Design review of the part shown in the three views and the two pictorial views. Dimensions are in mm from the part's minimum x, y and z. Coordinates: 2 decimals unless noted, no trailing zeros. Order: outer loops, then holes, each group sorted by start corner. A loop starts at its lowest first (then second) coordinate and runs counter-clockwise, first axis right, second up. Notation, with made-up numbers: (5.25, 38.5) -> (26.25, 38.5) arc R12 cw to (26.25, 54.5) -> close; hole circle Ø3 at (64.25, 88.25). An arc over 180 degrees is marked (long way). Answer as a JSON object with one key per item and string values. Group by question number.
1) Add section B-B, the plane z = 34. Write out the cut boundary in (x, y).
2) Add section A-A, the plane y = 7.5. Write out the cut boundary in (x, z).
3) Wall thickness on L1, parallel to Y at x = 40, z = 47.5; L2, parallel to X at y = 13, z = 33; L3, parallel to X at y = 4, z = 5.5 (1 decimal): over which ranges is each line inside the solid? List them lowest first.
4) Add section D-D, the plane y = 13.5. Write out the cut boundary in (x, z), then the cut area to 3 significant figures.
5) Add section C-C, the plane x = 44. Write out the cut boundary in (y, z), then the cut area to 3 significant figures.
6) For pin 1 (1.5 mm diameter, centred on x = 34.5, y = 12.5, fed in from +Z); pin 2 (1.5 mm diameter, centred on x = 31.5, y = 12, fed in from -Z); pin 3 (2.5 mm diameter, centred on y = 13, z = 27.5, fed in from -X), all flat-tipped, find the tip position at first contact; note any pin that passes through.
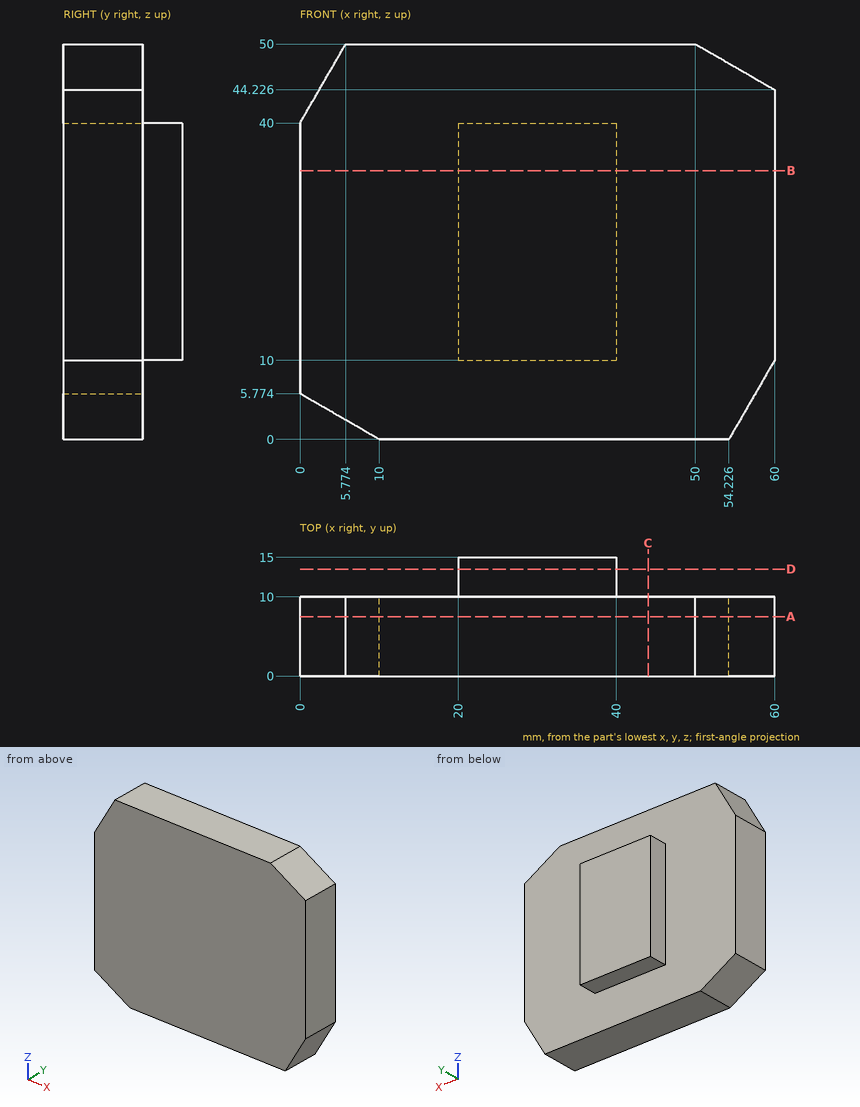
Output values:
{
 "1": {"outline": "(0, 0) -> (60, 0) -> (60, 10) -> (40, 10) -> (40, 15) -> (20, 15) -> (20, 10) -> (0, 10) -> close"},
 "2": {"outline": "(0, 5.77) -> (10, 0) -> (54.23, 0) -> (60, 10) -> (60, 44.23) -> (50, 50) -> (5.77, 50) -> (0, 40) -> close"},
 "3": {"L1": "y = 0 to 10", "L2": "x = 20 to 40", "L3": "x = 0.5 to 57.4"},
 "4": {"outline": "(20, 10) -> (40, 10) -> (40, 40) -> (20, 40) -> close", "area": "600 mm²"},
 "5": {"outline": "(0, 0) -> (10, 0) -> (10, 50) -> (0, 50) -> close", "area": "500 mm²"},
 "6": {"pin 1": "stops at z = 40", "pin 2": "stops at z = 10", "pin 3": "stops at x = 20"}
}
